from build123d import *

# Parameters (mm, degrees)
F0_W     = 481.25
F0_H     = 350
F1_DEPTH = 401.25
F2_W     = 480
F2_H     = 400
F3_DEPTH = 350.001
F5_DEPTH = 481.251
F7_DEPTH = 401.251
F8_SCALE = 2.54


with BuildPart() as f1:
    # F0 (on Front) → F1 (new body)
    with BuildSketch(Plane.XZ):
        with Locations((240.625, 175)):
            Rectangle(F0_W, F0_H)
    extrude(amount=-F1_DEPTH)

    # F2 (on face) → F3 (cut, through all)
    with BuildSketch(Plane.XY.offset(350)):
        with Locations((240.625, 200.625)):
            Rectangle(F2_W, F2_H)
    extrude(amount=-F3_DEPTH, mode=Mode.SUBTRACT)

    # F4 (on face) → F5 (cut, through all)
    with BuildSketch(Plane(origin=(0, 0, 0), x_dir=(0, -1, 0), z_dir=(-1, 0, 0))):
        Polygon((-346.25, 50), (-346.25, 0), (-346.25, -50), (-55, -50), (-55, 50), align=None)
    extrude(amount=-F5_DEPTH, mode=Mode.SUBTRACT)

    # F6 (on face) → F7 (cut, through all)
    with BuildSketch(Plane.XZ):
        Polygon((75, 50), (75, 0), (75, -50), (406.25, -50), (406.25, 50), align=None)
    extrude(amount=-F7_DEPTH, mode=Mode.SUBTRACT)


with BuildPart() as f1_1:
    # F8: moved
    add(f1.part.scale(F8_SCALE).moved(Location((-741.125, 0, 0))))


solid = f1_1.part
Here's how the part is built. I have some questions about the finished solid (model axes, mm). A direction names the side the tool comes from. Give positions to 0.01 mm unless a question says otherwise; leave off trailing zeros. Write each loop counter-clockwise with the first axis right and the second up, starting at its lowest first coordinate (ties: lowest second). Pieces come first, ordered by that corner, then holes. Notation, with made-up numbers: (23.25, 75.5) -> (42.25, 75.5) arc R13 cw to (42.25, 100.5) -> close; hole circle Ø3 at (37, -0.5). An arc over 180 degrees is marked (long way). Use one line per item in the form item = value. Start each with the question number.
1. Thinking about a two-plate mould opening in Y: for faces 1 (the face through (-138, 1.588, 451)), 2 (the face through (-138, 1019.175, 451)), 3 (the face through (-741.125, 502, 438)), which applies, +Y half, -Y half, draft (parallel to the pull), parting line (faces both ways), or undercut?
2. If I drill on L1, parallel to Y at x = -240.5, z = 849 (1 decimal), over which ranges is the centre line in solid material (lowest first)?
3. Will these pins go through, and if not, where does the flat tip stop? pin 1 Ø1.3 at (x, z) = (-740, 77.5) entering from -Y; pin 2 Ø0.5 at (x, y) = (-740.5, 689) entering from -Z.
4. On a 3-axis mill with a long thin cutter (end or side, diameter ignored), from which of +Z, -Z, +X, -X, +Y, -Y can I reach the whole of each face in a straight line? I mean faces 4 (the face through (-138, 0, 451)), 5 (the face through (-138, 1017.588, 451)). Say none if no direction works.
5. Imagine slicing it at A-A on x = -635.5. List the corners of the cut face in (y, z) for me (1 decimal), plus the area to 3 significant figures.
Entries:
q1.face_1 = undercut
q1.face_2 = +Y half
q1.face_3 = draft
q2.L1 = 0 to 1.6, 1017.6 to 1019.2
q3.pin_1 = 0
q3.pin_2 = 127
q4.face_4 = +Z, -Z, +X, -X, -Y
q4.face_5 = +Z, -Z
q5.outline = (0, 0) -> (1.6, 0) -> (1.6, 889) -> (0, 889) -> close; (1017.6, 0) -> (1019.2, 0) -> (1019.2, 889) -> (1017.6, 889) -> close
q5.area = 2,820 mm²
